Design review of the part built by this model. Coordinates are the model's own, in mm. Face numbers are marked on the shaded views. A direction names the side the tool comes from. Round coordinates to 2 decimals unless told otherwise and drop trailing zeros. Order: outer loops, then holes, each group sorted by start corner. A loop starts at its lowest first (then second) coordinate and runs counter-clockwise, first axis right, second up. Notation, with made-up numbers: (42, 33.25) - (86, 33.25) arc R32 ccw to (86, 66.25) - close; hole circle Ø7 at (53.25, 1.25). An arc over 180 degrees is marked (long way). Answer as a JSON object with one key per item and string values. Group by question number.
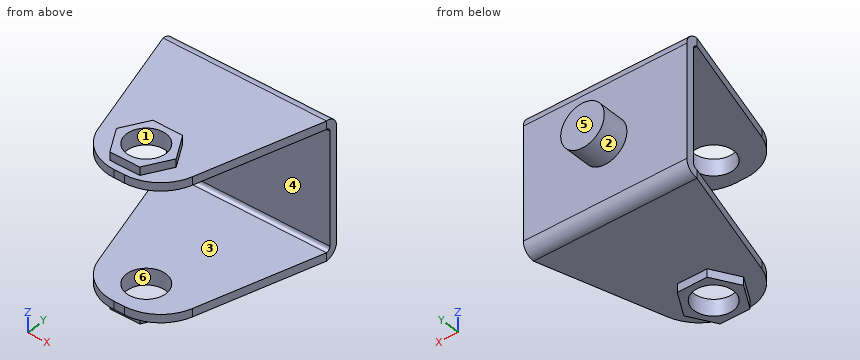
from build123d import *

# Parameters (mm, degrees)
SKETCH1_W                      = 30
SKETCH1_H                      = 22
BASE_FLANGE1_DEPTH             = 1.5
EDGE_FLANGE1_STRIP_W           = 7.4732
EDGE_FLANGE1_STRIP_H           = 1.5
EDGE_FLANGE1_STRIP_CUT_DEPTH   = 30
EDGE_FLANGE1_STRIP_2_W         = 7.4732
EDGE_FLANGE1_STRIP_2_H         = 1.5
EDGE_FLANGE1_STRIP_CUT_2_DEPTH = 30
EDGE_FLANGE1_DEPTH             = 30
EDGE_FLANGE1_BEND_DEPTH        = 30
CUT_EXTRUDE1_DEPTH             = 42.833001327
FILLET1_R                      = 8
SKETCH12_R                     = 3.6
CUT_EXTRUDE2_DEPTH             = 42.833001327
BOSS_EXTRUDE1_START            = 1.5
SKETCH13_R                     = 3.6
BOSS_EXTRUDE1_DEPTH            = 1.5
SKETCH14_R                     = 6
BOSS_EXTRUDE2_DEPTH            = 1
SKETCH15_R                     = 10
BOSS_EXTRUDE3_DEPTH            = 4
FILLET2_R                      = 2
SKETCH16_R                     = 4
BOSS_EXTRUDE4_DEPTH            = 5
CUT_EXTRUDE4_START             = -10
SKETCH17_R                     = 10.163794577
SKETCH17_R_2                   = 4
CUT_EXTRUDE4_DEPTH             = 10
CUT_EXTRUDE5_START             = -5
SKETCH18_R                     = 4
CUT_EXTRUDE5_DEPTH             = 5


# Sheet-metal steps are written as plain solids
with BuildPart() as part:
    # Sketch1 → Base-Flange1 (new body)
    with BuildSketch(Plane(origin=(0, 0, 0), x_dir=(1, 0, 0), z_dir=(0, 1, 0))):
        Rectangle(SKETCH1_W, SKETCH1_H)
    extrude(amount=-BASE_FLANGE1_DEPTH)

    # Edge-Flange1 strip (across the edge) → Edge-Flange1 strip cut (cut)
    with BuildSketch(Plane(origin=(15, -1.5, 11), x_dir=(0, 0, -1), z_dir=(-1, 0, 0))):
        with Locations((-3, -0.75)):
            Rectangle(EDGE_FLANGE1_STRIP_W, EDGE_FLANGE1_STRIP_H)
    extrude(amount=EDGE_FLANGE1_STRIP_CUT_DEPTH, mode=Mode.SUBTRACT)

    # Edge-Flange1 strip 2 (across the edge) → Edge-Flange1 strip cut 2 (cut)
    with BuildSketch(Plane(origin=(-15, -1.5, -11), x_dir=(0, 0, 1), z_dir=(1, 0, 0))):
        with Locations((-3, -0.75)):
            Rectangle(EDGE_FLANGE1_STRIP_2_W, EDGE_FLANGE1_STRIP_2_H)
    extrude(amount=EDGE_FLANGE1_STRIP_CUT_2_DEPTH, mode=Mode.SUBTRACT)

    # Edge-Flange1 section (across the edge) → Edge-Flange1 (add)
    with BuildSketch(Plane(origin=(15, -1.5, 11), x_dir=(0, 0, -1), z_dir=(-1, 0, 0))):
        with BuildLine():
            Line((-1.5, 0.7366), (-1.5, 28.5))
            Line((-1.5, 28.5), (0, 28.5))
            Line((0, 28.5), (0, 0.7366))
            ThreePointArc((0, 0.7366), (0.215745145, 0.215745145), (0.7366, 0))
            Line((0.7366, 0), (0.7366, -1.5))
            ThreePointArc((0.7366, -1.5), (-0.844915027, -0.844915027), (-1.5, 0.7366))
        make_face()
    extrude(amount=EDGE_FLANGE1_DEPTH)

    # Edge-Flange1 section 2 (across the edge) → Edge-Flange1 bend (add)
    with BuildSketch(Plane(origin=(-15, -1.5, -11), x_dir=(0, 0, 1), z_dir=(1, 0, 0))):
        with BuildLine():
            Line((-1.5, 0.7366), (-1.5, 28.5))
            Line((-1.5, 28.5), (0, 28.5))
            Line((0, 28.5), (0, 0.7366))
            ThreePointArc((0, 0.7366), (0.215745145, 0.215745145), (0.7366, 0))
            Line((0.7366, 0), (0.7366, -1.5))
            ThreePointArc((0.7366, -1.5), (-0.844915027, -0.844915027), (-1.5, 0.7366))
        make_face()
    extrude(amount=EDGE_FLANGE1_BEND_DEPTH)

    # Sketch11 → Cut-Extrude1 (cut, through all)
    with BuildSketch(Plane.XY.offset(12.5)):
        Polygon((-15, -2.2366), (-7, -30), (-15, -30), align=None)
        Polygon((15, -2.2366), (7, -30), (15, -30), align=None)
    extrude(amount=-CUT_EXTRUDE1_DEPTH, mode=Mode.SUBTRACT)

    # Fillet1
    fillet1_edges = [part.edges().sort_by_distance(p)[0] for p in [
        (7, -30, 11.75),
        (7, -30, -11.75),
        (-7, -30, 11.75),
        (-7, -30, -11.75),
    ]]
    fillet(fillet1_edges, radius=FILLET1_R)

    # Sketch12 → Cut-Extrude2 (cut, through all)
    with BuildSketch(Plane.XY.offset(12.5)):
        with Locations((0, -24)):
            Circle(SKETCH12_R)
    extrude(amount=-CUT_EXTRUDE2_DEPTH, mode=Mode.SUBTRACT)

    # Sketch13 → Boss-Extrude1 (add)
    with BuildSketch(Plane.XY.offset(12.5).offset(BOSS_EXTRUDE1_START)):
        Polygon((5.484827557, -24), (2.742413779, -19.25), (-2.742413779, -19.25), (-5.484827557, -24), (-2.742413779, -28.75), (2.742413779, -28.75), align=None)
        with Locations((0, -24)):
            Circle(SKETCH13_R, mode=Mode.SUBTRACT)
    boss_extrude1 = extrude(amount=-BOSS_EXTRUDE1_DEPTH)

    # Mirror1: Boss-Extrude1 across plane
    add(boss_extrude1.mirror(Plane.XY))

    # Sketch14 → Boss-Extrude2 (add)
    with BuildSketch(Plane(origin=(0, 0, 0), x_dir=(1, 0, 0), z_dir=(0, 1, 0))):
        with Locations(Location((0, 0, 0), (0, 0, 90))):
            Circle(SKETCH14_R)
    extrude(amount=BOSS_EXTRUDE2_DEPTH)

    # Sketch15 → Boss-Extrude3 (add)
    with BuildSketch(Plane(origin=(0, 1, 0), x_dir=(1, 0, 0), z_dir=(0, 1, 0))):
        with Locations(Location((0, 0, 0), (0, 0, 270))):
            Circle(SKETCH15_R)
    extrude(amount=BOSS_EXTRUDE3_DEPTH)

    # Fillet2
    fillet2_edges = [part.edges().sort_by_distance(p)[0] for p in [
        (0, 1, -10),
    ]]
    fillet(fillet2_edges, radius=FILLET2_R)

    # Sketch16 → Boss-Extrude4 (add)
    with BuildSketch(Plane(origin=(0, 5, 0), x_dir=(1, 0, 0), z_dir=(0, 1, 0))):
        with Locations(Location((0, 0, 0), (0, 0, 270))):
            Circle(SKETCH16_R)
    extrude(amount=BOSS_EXTRUDE4_DEPTH)

    # Sketch17 → Cut-Extrude4 (cut)
    with BuildSketch(Plane(origin=(0, 10, 0), x_dir=(1, 0, 0), z_dir=(0, 1, 0)).offset(CUT_EXTRUDE4_START)):
        Circle(SKETCH17_R)
        with Locations(Location((0, 0, 0), (0, 0, 270))):
            Circle(SKETCH17_R_2, mode=Mode.SUBTRACT)
    extrude(amount=CUT_EXTRUDE4_DEPTH, mode=Mode.SUBTRACT)

    # Sketch18 → Cut-Extrude5 (cut)
    with BuildSketch(Plane(origin=(0, 10, 0), x_dir=(1, 0, 0), z_dir=(0, 1, 0)).offset(CUT_EXTRUDE5_START)):
        with Locations(Location((0, 0, 0), (0, 0, 270))):
            Circle(SKETCH18_R)
    extrude(amount=CUT_EXTRUDE5_DEPTH, mode=Mode.SUBTRACT)


solid = part.part
1. Clearance check with flat-ended pins moving along their axes: P1, Ø5, axis at x = 4.5, z = 5, coming from the +Y side; P2, Ø6.5, axis at x = 0, y = -24, coming from the -Z side; P3, Ø1, axis at x = 5, z = 8.5, coming from the -Y side; P4, Ø3, axis at x = -8, z = 11, coming from the -Y side. State where each tip first meets the part, or that it passes through.
2. To check wall thickness, follow line 1 (Y direction, x = 0, z = -12.8); line 2 (Z direction, x = -3, y = -2.5); line 3 (Y direction, x = 13.5, z = -3.5). State the ranges of each line that lie inside material, in increasing order. Write a range as from..to.
3. Take a section at C-C, the plane y = -9. Give the boundary of the cut face in (x, z).
4. Take a section at A-A, the plane x = 0. Count the separate pieces of the cut face and the enclosed holes in it, then the cut area to 3 significant figures.
5. Mouldability with a two-part tool opening along Y and no side actions: class the marked faces 4, 5 and 6 as pulls with the +Y half, pulls with the -Y half, needs draft (parallel to the pull), parting line crosses it, or undercut.
6. Take a section at D-D, the plane x = -7. Give the boundary of the cut face in (y, z), then the cut area to 3 significant figures.
7. Tool access review of the marked faces 1, 2 and 3: name each direction out of +Z, -Z, +X, -X, +Y, -Y from which nothing blocks a thin tool from reaching the whole face with its end or side.
8. Take a section at B-B, the plane z = 0. Give the boundary of the cut face in (x, y).
Response values:
{
 "1": {"P1": "y = 0", "P2": "through", "P3": "y = -1.5", "P4": "y = -27.79"},
 "2": {"line 1": "-28.75..-27.6, -20.4..-19.25", "line 2": "-12.5..-11, 11..12.5", "line 3": "-1.5..0"},
 "3": {"outline": "(-13.05, -12.5) - (13.05, -12.5) - (13.05, -11) - (-13.05, -11) - close; (-13.05, 11) - (13.05, 11) - (13.05, 12.5) - (-13.05, 12.5) - close"},
 "4": {"separate pieces": "3", "enclosed holes": "0", "area": "146 mm2"},
 "5": {"face 4": "pulls with the -Y half", "face 5": "pulls with the +Y half", "face 6": "undercut"},
 "6": {"outline": "(-27.27, -12.5) - (-2.24, -12.5) arc R2.24 ccw to (0, -10.26) - (0, 10.26) arc R2.24 ccw to (-2.24, 12.5) - (-27.27, 12.5) - (-27.27, 11) - (-2.24, 11) arc R0.74 cw to (-1.5, 10.26) - (-1.5, -10.26) arc R0.74 cw to (-2.24, -11) - (-27.27, -11) - close", "area": "113 mm2"},
 "7": {"face 1": "+Z, -Z", "face 2": "+Y", "face 3": "+X, -X, -Y"},
 "8": {"outline": "(-15, -1.5) - (15, -1.5) - (15, 0) - (4, 0) - (4, 5) - (-4, 5) - (-4, 0) - (-15, 0) - close"}
}
